Model file for the job. Use its own axes, mm. A direction names the side the tool comes from. Give positions to 0.01 mm unless a question says otherwise; leave off trailing zeros. Loops run counter-clockwise (first coordinate to the right, second up) from the corner with the lowest first, then second, coordinate; pieces in that order, holes last. Notation, with made-up numbers: M 88,-39 L 107,-39 A6 cw 107,-33 Z; hole C -30,28 d7. An arc over 180 degrees is marked long. Answer in a Markdown table with one row per item.
```python
from build123d import *

# Parameters (mm, degrees)
SLOT_REACH = 11.649


with BuildPart() as part:
    # Sk1 → Body (revolve)
    with BuildSketch(Plane.XY, mode=Mode.PRIVATE) as body_sk:
        Polygon((-6.14, 0), (1.86, 0), (1.86, 2.77), (1.27, 2.77), (0, 1.5), (-6.14, 1.5), align=None)
    revolve(body_sk.sketch.rotate(Axis((0, 0, 0), (1, 0, 0)), 90), axis=Axis((0, 0, 0), (1, 0, 0)))

    # Slot: up to this cone (the profile starts inside it)
    slot_end = Plane(origin=(1.86, 0, 0), z_dir=(1, 0, 0)).offset(-1.764817835) * Cone(1.732e-06, 29.393897654, 16.970573723, align=(Align.CENTER, Align.CENTER, Align.MIN), mode=Mode.PRIVATE)
    # Sk2 → Slot (cut, up to the surface)
    with BuildSketch(Plane(origin=(1.86, 0, -1.86), x_dir=(0, 0, 1), z_dir=(-1, 0, 0)), mode=Mode.PRIVATE) as slot_sk1:
        Polygon((1.86, 1.154700538), (0.86, 0.577350269), (0.86, -0.577350269), (1.86, -1.154700538), (2.86, -0.577350269), (2.86, 0.577350269), align=None)
    slot_tool1 = extrude(slot_sk1.sketch, amount=SLOT_REACH, mode=Mode.PRIVATE) & slot_end
    add(slot_tool1.solids().sort_by_distance((1.86, 0, 0))[0], mode=Mode.SUBTRACT)


solid = part.part
```
(1) Which spindle directions (+Z, -Z, +X, -X, +Y, -Y) get a long thin tool onto all of the face, cutting with end or side? Do faces 1 (the flat face through (1, 0, 1)), 2 (the cylindrical face through (1.561, 1.686, -2.198)). Say none if no direction does.
Established:
| item | result |
|---|---|
| face 1 | +X |
| face 2 | +X, -X |
(2) Saw through at A-A, the plane x = 0.25. Give the cut face in (y, z).
Established:
| item | result |
|---|---|
| outline | C 0,0 d3.5; hole C 0,0 d0.54 |
(3) Mould opens along Z. For faces 3 (the cylindrical face through (-3.11, -0.45, 1.43)), 4 (the flat face through (1.86, 0, -1.2)), 5 (the flat face through (1, 0, -1)) say: pulls with the +Z half, pulls with the -Z half, needs draft (parallel to the pull), parting line crosses it, or undercut.
Established:
| item | result |
|---|---|
| face 3 | parting line crosses it |
| face 4 | needs draft |
| face 5 | undercut |
(4) Saw through at B-B, the plane x = -3. Give the cut face in (y, z), and give its area (3 significant figures).
Established:
| item | result |
|---|---|
| outline | C 0,0 d3 |
| area | 7.07 mm2 |
(5) Wall check: L1, parallel to Y at x = 1.5, z = 0.8; L2, parallel to Y at x = -3.5, z = -0.8; L3, parallel to Y at x = -1.5, z = 1.2. Give the ranges that are in metal, low to high.
Established:
| item | result |
|---|---|
| L1 | y = -2.65 to -0.69, 0.69 to 2.65 |
| L2 | y = -1.27 to 1.27 |
| L3 | y = -0.9 to 0.9 |
(6) Flat gauge pins, fed straight in: P1, Ø1.5, axis at x = 0, y = 0.5, coming from the -Z side; P2, Ø3, axis at x = -3.5, y = 0.5, coming from the +Z side; P3, Ø0.9, axis at x = 1, y = 0, coming from the -Z side. Where does each tip first touch, or does it go through?
Established:
| item | result |
|---|---|
| P1 | stops at z = -2.21 |
| P2 | stops at z = 1.5 |
| P3 | stops at z = -2.77 |
